Part model, mm, in its own coordinate system. Face numbers are marked on the shaded views. A direction names the side the tool comes from. Coordinates: 2 decimals unless noted, no trailing zeros. Write each loop counter-clockwise with the first axis right and the second up, starting at its lowest first coordinate (ties: lowest second). Pieces come first, ordered by that corner, then holes. Notation, with made-up numbers: (41.5, 51) -> (52.5, 51) arc R31 cw to (52.5, 86) -> close; hole circle Ø11 at (8.25, -26.75). An arc over 180 degrees is marked (long way). Write item = value, one per line. Start each with the question number.
Q1. Band-saw the part on B-B, the plane y = -29.5. List the corners of the cut face in (x, z).
Q2. Band-saw the part on A-A, the plane z = -119. List the corners of the cut face in (x, y).
Q3. Probe line 1 (X direction, y = -475, z = -1); line 2 (X direction, y = 475, z = -192.75); line 3 (X direction, y = 299, z = -51). List the from-to ranges inside material, lowest first.
Q4. Tool access for the marked faces 5 and 6: list every direction of +Z, -Z, +X, -X, +Y, -Y with a clear straight run to the whole face (end or side of a thin tool).
Q5. Pull direction X, two halves, no side cores. Call the marked faces 1, 2, 3 and 4: released by +X, released by -X, zero draft, split by the parting line, or undercut.
Q6. Band-saw the part on C-C, the plane x = 85. List the corners of the cut face in (y, z).
Q7. Pin check, flat tip, straight feed: P1, Ø19, axis at x = 160.45, y = -475, coming from the -Z side. Stop position of the tip, or through.
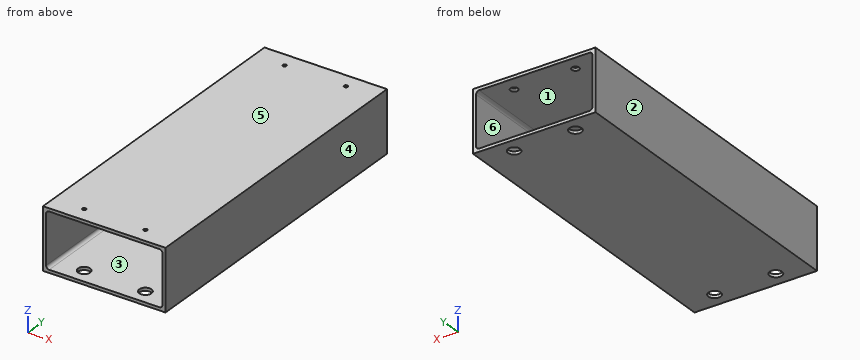
from build123d import *

# Parameters (mm, degrees)
F0_W     = 400
F0_H     = 200
F1_DEPTH = 525
F2_R     = 6
F3_DEPTH = 200.001
F4_R     = 20
F5_DEPTH = 25
F6_SIZE  = 6


with BuildPart() as f1:
    # F0 (on Front) → F1 (new body, symmetric)
    with BuildSketch(Plane.XZ):
        with Locations((60.4516596433, -100)):
            Rectangle(F0_W, F0_H)
        with BuildLine():
            ThreePointArc((-129.5483403567, -20), (-126.6194081686, -12.9289321881), (-119.5483403567, -10))
            Line((-119.5483403567, -10), (240.4516596433, -10))
            ThreePointArc((240.4516596433, -10), (247.5227274551, -12.9289321881), (250.4516596433, -20))
            Line((250.4516596433, -20), (250.4516596433, -180))
            ThreePointArc((250.4516596433, -180), (247.5227274551, -187.0710678119), (240.4516596433, -190))
            Line((240.4516596433, -190), (-119.5483403567, -190))
            ThreePointArc((-119.5483403567, -190), (-126.6194081686, -187.0710678119), (-129.5483403567, -180))
            Line((-129.5483403567, -180), (-129.5483403567, -20))
        make_face(mode=Mode.SUBTRACT)
    extrude(amount=F1_DEPTH, both=True)

    # F2 (on face) → F3 (cut, through all)
    with BuildSketch(Plane.XY):
        with Locations((-39.5483403567, -475)):
            Circle(F2_R)
        with Locations((160.4516596433, -475)):
            Circle(F2_R)
        with Locations((-39.5483403567, 475)):
            Circle(F2_R)
        with Locations((160.4516596433, 475)):
            Circle(F2_R)
    extrude(amount=-F3_DEPTH, mode=Mode.SUBTRACT)

    # F4 (on face) → F5 (cut)
    with BuildSketch(Plane(origin=(0, 0, -200), x_dir=(1, 0, 0), z_dir=(0, 0, -1))):
        with Locations((-39.5483403567, 475)):
            Circle(F4_R)
        with Locations((160.4516596433, 475)):
            Circle(F4_R)
        with Locations((-39.5483403567, -475)):
            Circle(F4_R)
        with Locations((160.4516596433, -475)):
            Circle(F4_R)
    extrude(amount=-F5_DEPTH, mode=Mode.SUBTRACT)

    # F6
    f6_edges = [f1.edges().sort_by_distance(p)[0] for p in [
        (-45.54834, -475, -10),
        (154.45166, -475, -10),
        (-45.54834, 475, -10),
        (154.45166, 475, -10),
    ]]
    chamfer(f6_edges, length=F6_SIZE)


solid = f1.part
Ans:
q1.outline = (-139.55, -200) -> (260.45, -200) -> (260.45, 0) -> (-139.55, 0) -> close; hole (-129.55, -180) arc R10 ccw to (-119.55, -190) -> (240.45, -190) arc R10 ccw to (250.45, -180) -> (250.45, -20) arc R10 ccw to (240.45, -10) -> (-119.55, -10) arc R10 ccw to (-129.55, -20) -> close
q2.outline = (-139.55, -525) -> (-129.55, -525) -> (-129.55, 525) -> (-139.55, 525) -> close; (250.45, -525) -> (260.45, -525) -> (260.45, 525) -> (250.45, 525) -> close
q3.line_1 = -139.55 to -45.55, -33.55 to 154.45, 166.45 to 260.45
q3.line_2 = -139.55 to -59.55, -19.55 to 140.45, 180.45 to 260.45
q3.line_3 = -139.55 to -129.55, 250.45 to 260.45
q4.face_5 = +Z, +X, -X, +Y, -Y
q4.face_6 = +Y, -Y
q5.face_1 = undercut
q5.face_2 = released by -X
q5.face_3 = undercut
q5.face_4 = released by +X
q6.outline = (-525, -200) -> (525, -200) -> (525, -190) -> (-525, -190) -> close; (-525, -10) -> (525, -10) -> (525, 0) -> (-525, 0) -> close
q7.P1 = -7.5
